Could you check a few things on this model? Use its own coordinates, in mm. A direction names the side the tool comes from. Give positions to 0.01 mm unless a question says otherwise; leave off trailing zeros. Write each loop counter-clockwise with the first axis right and the second up, starting at its lowest first coordinate (ties: lowest second). Pieces come first, ordered by that corner, then holes. Notation, with made-up numbers: (59, 6.25) - (79, 6.25) arc R26 cw to (79, 32.25) - close; hole circle Ø4 at (77.25, 89). An arc over 180 degrees is marked (long way). Write item = value, one per line.
from build123d import *

# Parameters (mm, degrees)
EXTRUDE1_DEPTH      = 10.3
EXTRUDE1_DEPTH_BACK = 10.3
SKETCH1_W           = 11
SKETCH1_H           = 55
EXTRUDE2_DEPTH      = 6
SKETCH5_R           = 5.5
EXTRUDE4_DEPTH      = 69.744308855
SKETCH_1_R          = 2.8
CUT_EXTRUDE_1_DEPTH = 76.545350618
FILLET2_R           = 1.5
SKETCH_4_R          = 6.7
CUT_EXTRUDE_2_DEPTH = 9
SKETCH_5_R          = 12.5
CUT_EXTRUDE_3_DEPTH = 3.4
SKETCH_6_R          = 0.9
CUT_EXTRUDE_4_DEPTH = 7
CHAMFER_1_SIZE      = 1


with BuildPart() as part:
    # Sketch1 → Extrude1 (new, two sides: drawn at the far end of the back side and taken through both)
    with BuildSketch(Plane(origin=(0, 0, 0), x_dir=(0, 0, -1), z_dir=(1, 0, 0)).offset(-EXTRUDE1_DEPTH_BACK)):
        with Locations((0, 37.8)):
            Rectangle(SKETCH1_W, SKETCH1_H)
    extrude(amount=EXTRUDE1_DEPTH + EXTRUDE1_DEPTH_BACK)

    # Sketch2 → Extrude2 (add)
    with BuildSketch(Plane(origin=(10.3, 0, 0), x_dir=(0, 0, -1), z_dir=(1, 0, 0))):
        with BuildLine():
            Line((-19.5, 10), (-19.5, -10))
            Line((-19.5, -10), (5.5, -10))
            Line((5.5, -10), (5.5, 17))
            Line((5.5, 17), (5.5, 65.3))
            Line((5.5, 65.3), (-5.5, 65.3))
            Line((-5.5, 65.3), (-5.5, 17))
            ThreePointArc((-5.5, 17), (-7.550252532, 12.050252532), (-12.5, 10))
            Line((-12.5, 10), (-19.5, 10))
        make_face()
    extrude2 = extrude(amount=EXTRUDE2_DEPTH)

    # Mirror2: Extrude2 across plane
    add(extrude2.mirror(Plane(origin=(0, 0, 0), x_dir=(0, 0, 1), z_dir=(1, 0, 0))))

    # Sketch5 → Extrude4 (cut, through all)
    with BuildSketch(Plane.XY.offset(5.5)):
        with Locations((0, 44)):
            Circle(SKETCH5_R)
    extrude(amount=-EXTRUDE4_DEPTH, mode=Mode.SUBTRACT)

    # Эскиз1 → Вырез-Вытянуть1 (cut, through all)
    with BuildSketch(Plane(origin=(16.3, 0, 0), x_dir=(0, 0, -1), z_dir=(1, 0, 0))):
        with Locations((-13, 0)):
            Circle(SKETCH_1_R)
        with Locations(Location((-1, 0, 0), (0, 0, 180))):
            Circle(SKETCH_1_R)
    extrude(amount=-CUT_EXTRUDE_1_DEPTH, mode=Mode.SUBTRACT)

    # Fillet2
    fillet2_edges = [part.edges().sort_by_distance(p)[0] for p in [
        (13.3, -10, 19.5),
        (13.3, -10, -5.5),
        (13.3, 10, 19.5),
        (-13.3, -10, -5.5),
        (-13.3, -10, 19.5),
        (-13.3, 10, 19.5),
        (0, 65.3, 5.5),
        (0, 65.3, -5.5),
    ]]
    fillet(fillet2_edges, radius=FILLET2_R)

    # Эскиз4 → Вырез-Вытянуть2 (cut)
    with BuildSketch(Plane.XY.offset(5.5)):
        with Locations((0, 44)):
            Circle(SKETCH_4_R)
    extrude(amount=-CUT_EXTRUDE_2_DEPTH, mode=Mode.SUBTRACT)

    # Эскиз5 → Вырез-Вытянуть3 (cut)
    with BuildSketch(Plane.XY.offset(5.5)):
        with Locations((0, 44)):
            Circle(SKETCH_5_R)
    extrude(amount=-CUT_EXTRUDE_3_DEPTH, mode=Mode.SUBTRACT)

    # Эскиз6 → Вырез-Вытянуть4 (cut)
    with BuildSketch(Plane.XY.offset(2.1)):
        with Locations((0, 53.5)):
            Circle(SKETCH_6_R)
        with Locations((9.5, 44)):
            Circle(SKETCH_6_R)
        with Locations((0, 34.5)):
            Circle(SKETCH_6_R)
        with Locations((-9.5, 44)):
            Circle(SKETCH_6_R)
    extrude(amount=-CUT_EXTRUDE_4_DEPTH, mode=Mode.SUBTRACT)

    # Фаска1
    chamfer_1_edges = [part.edges().sort_by_distance(p)[0] for p in [
        (-5.5, 44, -5.5),
    ]]
    chamfer(chamfer_1_edges, length=CHAMFER_1_SIZE)


solid = part.part
1. If we section it at A-A, the plane x = 0: Please give me the cut outline in (y, z), and give its area (3 significant figures).
Filled sheet:
outline = (10.3, -5.5) - (37.5, -5.5) - (38.5, -4.5) - (38.5, -3.5) - (37.3, -3.5) - (37.3, 2.1) - (35.4, 2.1) - (35.4, -4.9) - (33.6, -4.9) - (33.6, 2.1) - (31.5, 2.1) - (31.5, 5.5) - (10.3, 5.5) - close; (49.5, -4.5) - (50.5, -5.5) - (63.8, -5.5) arc R1.5 ccw to (65.3, -4) - (65.3, 4) arc R1.5 ccw to (63.8, 5.5) - (56.5, 5.5) - (56.5, 2.1) - (54.4, 2.1) - (54.4, -4.9) - (52.6, -4.9) - (52.6, 2.1) - (50.7, 2.1) - (50.7, -3.5) - (49.5, -3.5) - close
area = 396 mm2
2. If we section it at C-C, the plane y = 7.5: Please give me the cut outline in (x, z), and give its area (3 significant figures).
Filled sheet:
outline = (-16.3, -5.5) - (-10.3, -5.5) - (-10.3, 19.5) - (-16.3, 19.5) - close; (10.3, -5.5) - (16.3, -5.5) - (16.3, 19.5) - (10.3, 19.5) - close
area = 300 mm2
3. Which directions (+Z, -Z, +X, -X, +Y, -Y) give clear straight access to the entire face, cutting with the end or side of a thin tool? Please do faces 1 (the face through (-2.71, 31.797, 3.824)), 2 (the face through (13.34, -9.55, -5.07)), 3 (the face through (-13, 10, 15)).
Filled sheet:
face_1 = +Z
face_2 = -Z, +X, -X, -Y
face_3 = +Z, +X, -X, +Y
4. Thinking about a two-plate mould opening in Z: for faces 4 (the face through (-6, 44, -5)), 5 (the face through (-5, 47, -3.5)), 6 (the face through (13.3, -0.1, -1.8)), which applies, pulls with the +Z half, pulls with the -Z half, needs draft (parallel to the pull), parting line crosses it, or undercut?
Filled sheet:
face_4 = pulls with the -Z half
face_5 = pulls with the +Z half
face_6 = undercut
5. For pin 1 (0.5 mm diameter, centred on x = 0, y = 35, fed in from +Z); pin 2 (1.4 mm diameter, centred on x = -9, y = 43.5, fed in from +Z); pin 3 (3 mm diameter, centred on x = 5, y = 13, fed in from +Z); pin 4 (6.5 mm diameter, centred on y = 0, z = 13, fed in from -X), each with a flat end and sliding along its axis, tell me the tip position at first contact or that it passes through.
Filled sheet:
pin_1 = -4.9
pin_2 = 2.1
pin_3 = 5.5
pin_4 = -16.3
6. If we section it at D-D, the plane z = 6.5: Please give me the cut outline in (x, y), and give its area (3 significant figures).
Filled sheet:
outline = (-16.3, -10) - (-10.3, -10) - (-10.3, 13.39) - (-16.3, 13.39) - close; (10.3, -10) - (16.3, -10) - (16.3, 13.39) - (10.3, 13.39) - close
area = 281 mm2
7. If we section it at B-B, the plane z = -0.75: Please give me the cut outline in (x, y).
Filled sheet:
outline = (-16.3, -10) - (-10.3, -10) - (-10.3, -2.19) - (-16.3, -2.19) - close; (-16.3, 2.19) - (-10.3, 2.19) - (-10.3, 10.3) - (10.3, 10.3) - (10.3, 2.19) - (16.3, 2.19) - (16.3, 65.3) - (-16.3, 65.3) - close; (10.3, -10) - (16.3, -10) - (16.3, -2.19) - (10.3, -2.19) - close; hole circle Ø1.8 at (-9.5, 44); hole circle Ø13.4 at (0, 44); hole circle Ø1.8 at (0, 34.5); hole circle Ø1.8 at (0, 53.5); hole circle Ø1.8 at (9.5, 44)
8. I need wall thicknesses on line 1 (Y direction, x = 0, z = 0.5); line 2 (Y direction, x = 13.15, z = 13); line 3 (X direction, y = -6, z = 12.25). Which ranges of each line are inside material? Lowest first, please.
Filled sheet:
line_1 = 10.3 to 33.6, 35.4 to 37.3, 50.7 to 52.6, 54.4 to 65.3
line_2 = -10 to -2.8, 2.8 to 10
line_3 = -16.3 to -10.3, 10.3 to 16.3
